Here's how the part is built. I have some questions about the finished solid (model axes, mm). Face numbers are marked on the shaded views. Give positions to 0.01 mm unless a question says otherwise; leave off trailing zeros. Loops run counter-clockwise (first coordinate to the right, second up) from the corner with the lowest first, then second, coordinate; pieces in that order, holes last. Notation, with made-up numbers: (52.25, -13.75) -> (99.25, -13.75) arc R30 cw to (99.25, 22.25) -> close; hole circle Ø5 at (70.25, 0). An arc over 180 degrees is marked (long way). Answer in a Markdown table with one row per item. Add a question column.
Item 1: If we section it at A-A (y = 6): Give the number of separate pieces and of enclosed holes in the cut face, then the cut area to 3 significant figures.
Item 2: If we section it at C-C (z = 19): Write out the boundary of the cut face in (x, y), then the cut area to 3 significant figures.
Item 3: If we section it at D-D (x = 0): Write out the boundary of the cut face in (y, z).
Item 4: If I drill on line 1 (X direction, y = 6, z = 28.8); line 2 (Y direction, x = -36, z = 29.2); line 3 (X direction, y = 4.5, z = 10.5), over which ranges is the centre line in solid material (lowest first)?
Item 5: If we section it at B-B (x = -36): Write out the boundary of the cut face in (y, z).
Item 6: We'd pull the mould along X, two halves only. Please class the marked faces 1, 2 and 3: released by +X, released by -X, zero draft, split by the parting line, or undercut.
Item 7: For P1, Ø1.2, axis at x = -13, z = 29, coming from the +Y side; P2, Ø3, axis at x = -5.5, y = -2, coming from the -Z side; P3, Ø12, axis at x = 21, z = 15, coming from the +Y side, each with a flat end and sliding along its axis, tell me the tip position at first contact or that it passes through.
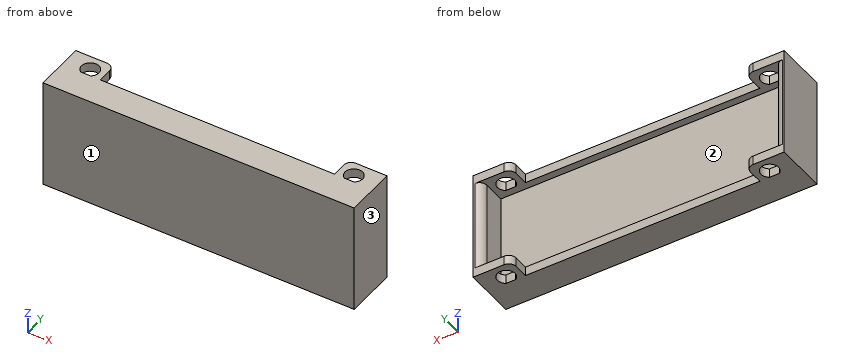
```python
from build123d import *

# Parameters (mm, degrees)
SKETCH1_W            = 85
SKETCH1_H            = 8
BOSS_EXTRUDE1_DEPTH  = 30
SKETCH2_W            = 80
SKETCH2_H            = 25
CUT_EXTRUDE1_DEPTH   = 2
BOSS_EXTRUDE3_DEPTH  = 6
M4_CLEARANCE_HOLE1_D = 4.8
FILLET1_R            = 2


with BuildPart() as part:
    # Sketch1 → Boss-Extrude1 (new body)
    with BuildSketch(Plane.XY):
        Rectangle(SKETCH1_W, SKETCH1_H)
    extrude(amount=BOSS_EXTRUDE1_DEPTH)

    # Sketch2 → Cut-Extrude1 (cut)
    with BuildSketch(Plane(origin=(0, 4, 0), x_dir=(1, 0, 0), z_dir=(0, 1, 0))):
        with Locations((0, -15)):
            Rectangle(SKETCH2_W, SKETCH2_H)
    extrude(amount=-CUT_EXTRUDE1_DEPTH, mode=Mode.SUBTRACT)

    # Sketch3 → Boss-Extrude3 (add)
    with BuildSketch(Plane(origin=(0, 4, 0), x_dir=(1, 0, 0), z_dir=(0, 1, 0))):
        Polygon((-32, 0), (-42.5, 0), (-42.5, -30), (-32, -30), (-32, -27.5), (-40, -27.5), (-40, -2.5), (-32, -2.5), align=None)
    extrude(amount=BOSS_EXTRUDE3_DEPTH)

    # M4 Clearance Hole1 (through all)
    with Locations(Plane.XY.offset(30)):
        with Locations((-36, 6)):
            Hole(M4_CLEARANCE_HOLE1_D / 2)

    # Fillet1
    fillet1_edges = [part.edges().sort_by_distance(p)[0] for p in [
        (-32, 10, 1.25),
        (-32, 10, 28.75),
        (-40, 10, 15),
    ]]
    fillet(fillet1_edges, radius=FILLET1_R)

    # Mirror1: part across plane


with BuildPart() as part_1:
    add(part.part)
    add(part.part.mirror(Plane(origin=(0, 0, 0), x_dir=(0, 0, 1), z_dir=(1, 0, 0))))


solid = part_1.part
```
Recorded:
| question | item | result |
|---|---|---|
| 1 | separate pieces | 6 |
| 1 | enclosed holes | 0 |
| 1 | area | 182 mm^2 |
| 2 | outline | (-42.5, -4) -> (42.5, -4) -> (42.5, 10) -> (42, 10) arc R2 ccw to (40, 8) -> (40, 2) -> (-40, 2) -> (-40, 8) arc R2 ccw to (-42, 10) -> (-42.5, 10) -> close |
| 2 | area | 548 mm^2 |
| 3 | outline | (-4, 0) -> (4, 0) -> (4, 2.5) -> (2, 2.5) -> (2, 27.5) -> (4, 27.5) -> (4, 30) -> (-4, 30) -> close |
| 4 | line 1 | x = -42.5 to -38.4, -33.6 to -32, 32 to 33.6, 38.4 to 42.5 |
| 4 | line 2 | y = -4 to 4, 8.4 to 10 |
| 4 | line 3 | x = -42.5 to -40, 40 to 42.5 |
| 5 | outline | (-4, 0) -> (4, 0) -> (4, 2.5) -> (2, 2.5) -> (2, 27.5) -> (4, 27.5) -> (4, 30) -> (-4, 30) -> close; (8.4, 0) -> (10, 0) -> (10, 2.5) -> (8.4, 2.5) -> close; (8.4, 27.5) -> (10, 27.5) -> (10, 30) -> (8.4, 30) -> close |
| 6 | face 1 | zero draft |
| 6 | face 2 | undercut |
| 6 | face 3 | released by +X |
| 7 | P1 | stops at y = 4 |
| 7 | P2 | stops at z = 0 |
| 7 | P3 | stops at y = 2 |
